Source: CAD feature listing. Evaluate the final solid. Frame: model axes, mm. A direction names the side the tool comes from. Round coordinates to 2 decimals unless told otherwise and drop trailing zeros. Order: outer loops, then holes, each group sorted by start corner. A loop starts at its lowest first (then second) coordinate and runs counter-clockwise, first axis right, second up. Notation, with made-up numbers: M 37.5,18 L 44.5,18 A14 cw 44.5,22 Z; hole C -35,9.5 d8. An arc over 180 degrees is marked long. Answer as CSV lines item,"result". Start each with the question number.
Item 1: Pull-direction query (X, two-part tool) for faces 4 (the face through (29.9, -10, 2.7)), 5 (the face through (14.52, 13.05, 5.07)), 6 (the face through (-37, -20, 5)), 7 (the face through (13.05, -14.52, 5.07)); classes: +X half, -X half, draft (parallel to the pull), parting line (faces both ways), or undercut.
Item 2: Set-up query: faces 1 (the face through (23, 7, 5)), 2 (the face through (-13.05, 14.52, 5.07)), 3 (the face through (-30.1, -10, 2.7)). Return all of +Z, -Z, +X, -X, +Y, -Y with unobstructed straight access to the full face (end or side cutting, diameter ignored); none if empty.
Item 3: First-contact query: P1, Ø4, axis at y = 15.5, z = 5.5, coming from the -X side; P2, Ø5, axis at y = 12.5, z = 6.5, coming from the +X side; P3, Ø5, axis at x = 26.5, z = 5, coming from the +Y side. Flat tips, straight axial feed; report the tip coordinate or a pass-through.
Item 4: Section query A-A on y = 0. Return the cut outline in (x, z), plus the area to 3 significant figures.
Item 5: Section query D-D on z = 9. Return the cut outline in (x, y).
Item 6: Section query B-B on x = 30. Return the cut outline in (y, z), plus the area to 3 significant figures.
Item 7: Section query C-C on z = 4. Return the cut outline in (x, y), plus the area to 3 significant figures.
Item 8: Line query: line 1 (Y direction, x = -13.5, z = 1.5); line 2 (Y direction, x = 0, z = 6.5); line 3 (X direction, y = -16, z = 4.5). Output: solid intervals per line, ascending. Write a range as [from, to].
from build123d import *

# Parameters (mm, degrees)
ESQUISSE1_R             = 13.15
BOSS_EXTRU_1_DEPTH      = 10
ENL_V_MAT_EXTRU_2_REACH = 67.406
ESQUISSE5_R             = 2.1
SKETCH1_R               = 2.25
CUT_EXTRUDE1_DEPTH      = 49.672374095
CIRPATTERN1_COUNT       = 4


with BuildPart() as part:
    # Esquisse1 → Boss.-Extru.1 (new body)
    with BuildSketch(Plane.XY):
        Polygon((-23, 23), (23, 23), (23, -10), (37, -10), (37, -30), (-37, -30), (-37, -10), (-23, -10), align=None)
        Circle(ESQUISSE1_R, mode=Mode.SUBTRACT)
    extrude(amount=BOSS_EXTRU_1_DEPTH)

    # Esquisse5 → Enlèv. mat.-Extru.2 (cut, up to next)
    with BuildSketch(Plane.XZ.offset(30), mode=Mode.PRIVATE) as enl_v_mat_extru_2_sk1:
        with Locations(Location((-30, 5, 0), (0, 0, 270))):
            Circle(ESQUISSE5_R)
    enl_v_mat_extru_2_tool1 = extrude(enl_v_mat_extru_2_sk1.sketch, amount=-ENL_V_MAT_EXTRU_2_REACH, mode=Mode.PRIVATE) & part.part
    # Esquisse5 → Enlèv. mat.-Extru.2 (cut, up to next)
    with BuildSketch(Plane.XZ.offset(30), mode=Mode.PRIVATE) as enl_v_mat_extru_2_sk2:
        with Locations(Location((30, 5, 0), (0, 0, 270))):
            Circle(ESQUISSE5_R)
    enl_v_mat_extru_2_tool2 = extrude(enl_v_mat_extru_2_sk2.sketch, amount=-ENL_V_MAT_EXTRU_2_REACH, mode=Mode.PRIVATE) & part.part
    add(enl_v_mat_extru_2_tool1.solids().sort_by_distance((-30, -30, 5))[0], mode=Mode.SUBTRACT)
    add(enl_v_mat_extru_2_tool2.solids().sort_by_distance((30, -30, 5))[0], mode=Mode.SUBTRACT)

    # Sketch1 → Cut-Extrude1 (cut, through all)
    with BuildSketch(Plane.XY.offset(10)):
        with Locations((12.374368671, 12.374368671)):
            Circle(SKETCH1_R)
    cut_extrude1 = extrude(amount=-CUT_EXTRUDE1_DEPTH, mode=Mode.SUBTRACT)

    # CirPattern1: Cut-Extrude1 ×4 about axis
    cirpattern1_axis = Axis((0, 0, 0), (0, 0, 1))
    for i in range(1, CIRPATTERN1_COUNT):
        add(cut_extrude1.rotate(cirpattern1_axis, i * 360 / CIRPATTERN1_COUNT), mode=Mode.SUBTRACT)


solid = part.part
Results:
1,face 4,"draft"
1,face 5,"undercut"
1,face 6,"-X half"
1,face 7,"undercut"
2,face 1,"+Z, -Z, +X, +Y"
2,face 2,"+Z, -Z"
2,face 3,"+Z, -Z, -X, +Y"
3,P1,"x = -23"
3,P2,"x = 23"
3,P3,"y = -10"
4,outline,"M -23,0 L -13.15,0 L -13.15,10 L -23,10 Z; M 13.15,0 L 23,0 L 23,10 L 13.15,10 Z"
4,area,"197 mm^2"
5,outline,"M -37,-30 L 37,-30 L 37,-10 L 23,-10 L 23,23 L -23,23 L -23,-10 L -37,-10 Z; hole C -12.37,-12.37 d4.5; hole C -12.37,12.37 d4.5; hole C 0,0 d26.3; hole C 12.37,-12.37 d4.5; hole C 12.37,12.37 d4.5"
6,outline,"M -30,0 L -10,0 L -10,2.9 L -30,2.9 Z; M -30,7.1 L -10,7.1 L -10,10 L -30,10 Z"
6,area,"116 mm^2"
7,outline,"M -37,-30 L -31.85,-30 L -31.85,-10 L -37,-10 Z; M -28.15,-30 L 28.15,-30 L 28.15,-10 L 23,-10 L 23,23 L -23,23 L -23,-10 L -28.15,-10 Z; M 31.85,-30 L 37,-30 L 37,-10 L 31.85,-10 Z; hole C -12.37,-12.37 d4.5; hole C -12.37,12.37 d4.5; hole C 0,0 d26.3; hole C 12.37,-12.37 d4.5; hole C 12.37,12.37 d4.5"
7,area,"2,240 mm^2"
8,line 1,"[-30, -14.32], [-10.43, 10.43], [14.32, 23]"
8,line 2,"[-30, -13.15], [13.15, 23]"
8,line 3,"[-37, -32.04], [-27.96, 27.96], [32.04, 37]"
